Geometry: final body of the model. Coordinates: model frame, mm. Round coordinates to 2 decimals unless told otherwise and drop trailing zeros. Loops run counter-clockwise (first coordinate to the right, second up) from the corner with the lowest first, then second, coordinate; pieces in that order, holes last. Notation, with made-up numbers: (53.25, -14.5) - (66.25, -14.5) arc R24 ccw to (66.25, 11.5) - close; hole circle Ø11 at (13.25, 58.25). An arc over 180 degrees is marked (long way). Answer as CSV lines item,"result".
from build123d import *

# Parameters (mm, degrees)
BOSS_EXTRUDE1_DEPTH = 12.7


with BuildPart() as part:
    # Sketch1 → Boss-Extrude1 (new, symmetric)
    with BuildSketch(Plane.XY):
        with BuildLine():
            Line((1.104550235, 1.012133813), (9.781107052, 0.253033453))
            ThreePointArc((9.781107052, 0.253033453), (10.012855938, -0.007594285), (9.765943465, -0.253904241))
            Line((9.765943465, -0.253904241), (0.521947944, -0.507808482))
            ThreePointArc((0.521947944, -0.507808482), (0.15375542, -0.364108195), (0, 0))
            ThreePointArc((0, 0), (0.329600349, 0.749073774), (1.104550235, 1.012133813))
        make_face()
    extrude(amount=BOSS_EXTRUDE1_DEPTH, both=True)


solid = part.part
(1) Section C-C (y = 0.55). Output: boundary loops of the cut face in (x, z).
Findings below:
outline,"(0.16, -12.7) - (6.39, -12.7) - (6.39, 12.7) - (0.16, 12.7) - close"
(2) Section A-A (z = 7.5). Output: boundary loops of the cut face in (x, y).
Findings below:
outline,"(0, 0) arc R0.51 ccw to (0.52, -0.51) - (9.77, -0.25) arc R0.25 ccw to (9.78, 0.25) - (1.1, 1.01) arc R1.02 ccw to start"
(3) Pin query (flat end, axial travel): P1, Ø3, axis at x = 8.5, z = 1.5, coming from the -Y side. Return the tip coordinate at first contact, or that it passes through.
Findings below:
P1,"y = -0.33"
(4) Section B-B (x = 7.75). Output: boundary loops of the cut face in (y, z).
Findings below:
outline,"(-0.31, -12.7) - (0.43, -12.7) - (0.43, 12.7) - (-0.31, 12.7) - close"
(5) Material intervals for line 1 along X through (y, z) = (-0.05, 6); line 2 along Y through (x, z) = (6.5, -2.5); line 3 along Y through (x, z) = (8.5, 4), sorted ascending.
Findings below:
line 1,"0 to 10.01"
line 2,"-0.34 to 0.54"
line 3,"-0.29 to 0.37"
